Part print with two shaded views. Sizes in mm from the minimum x, y, z corner. Round coordinates to 2 decimals unless told otherwise and drop trailing zeros. Write each loop counter-clockwise with the first axis right and the second up, starting at its lowest first coordinate (ties: lowest second). Pieces come first, ordered by that corner, then holes. Notation, with made-up numbers: (27, 35.5) -> (43, 35.5) arc R27 ccw to (43, 74.5) -> close; hole circle Ø6 at (72.25, -12). An arc over 180 degrees is marked (long way). Answer in a Markdown table with one row per item.
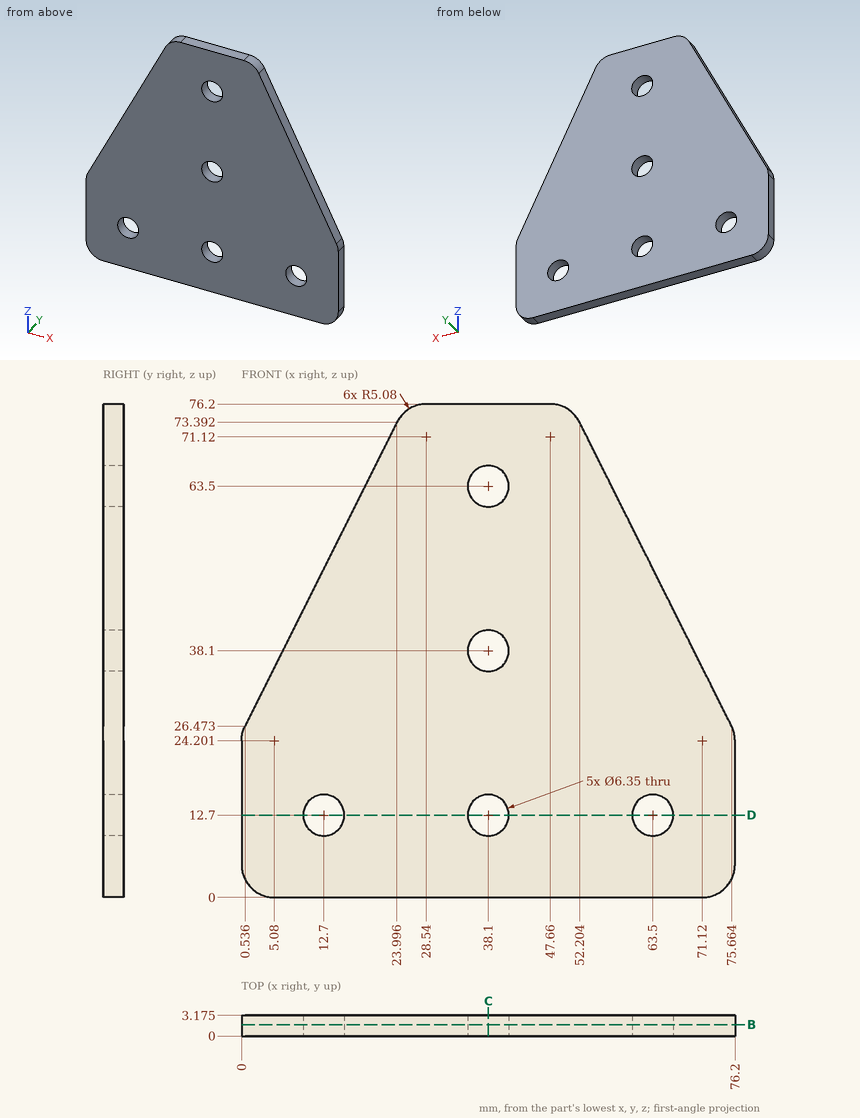
Q1. Saw through at B-B on y = 1.75. State how many separate pieces and enclosed holes the cut face has, plus the area to 3 significant figures.
A:
| item | result |
|---|---|
| separate pieces | 1 |
| enclosed holes | 5 |
| area | 4,340 mm² |
Q2. Wall check: line 1 (Z direction, x = 38.1, y = 2.5) (1 decimal); line 2 (Z direction, x = 12.7, y = 0.85) (1 decimal); line 3 (Z direction, x = 48, y = 1.8). Give the ranges that are in metal, low to high. Write a range as [from, to].
A:
| item | result |
|---|---|
| line 1 | [0, 9.5], [15.9, 34.9], [41.3, 60.3], [66.7, 76.2] |
| line 2 | [0, 9.5], [15.9, 50.8] |
| line 3 | [0, 76.19] |
Q3. Drop a flat-ended pin along its axis: P1, Ø4, axis at x = 38.1, z = 38.1, coming from the +Y side. Give the stop position or say it passes through.
A:
| item | result |
|---|---|
| P1 | through |
Q4. Saw through at C-C on x = 38.1. Write the cut outline in (y, z) (1 decimal).
A:
| item | result |
|---|---|
| outline | (0, 0) -> (3.2, 0) -> (3.2, 9.5) -> (0, 9.5) -> close; (0, 15.9) -> (3.2, 15.9) -> (3.2, 34.9) -> (0, 34.9) -> close; (0, 41.3) -> (3.2, 41.3) -> (3.2, 60.3) -> (0, 60.3) -> close; (0, 66.7) -> (3.2, 66.7) -> (3.2, 76.2) -> (0, 76.2) -> close |
Q5. Saw through at D-D on z = 12.7. Write the cut outline in (x, y) (1 decimal).
A:
| item | result |
|---|---|
| outline | (0, 0) -> (9.5, 0) -> (9.5, 3.2) -> (0, 3.2) -> close; (15.9, 0) -> (34.9, 0) -> (34.9, 3.2) -> (15.9, 3.2) -> close; (41.3, 0) -> (60.3, 0) -> (60.3, 3.2) -> (41.3, 3.2) -> close; (66.7, 0) -> (76.2, 0) -> (76.2, 3.2) -> (66.7, 3.2) -> close |
